Verification items for the finished model (mm, model axes). A direction names the side the tool comes from. Give positions to 0.01 mm unless a question says otherwise; leave off trailing zeros. Order: outer loops, then holes, each group sorted by start corner. A loop starts at its lowest first (then second) coordinate and runs counter-clockwise, first axis right, second up.
from build123d import *

# Parameters (mm, degrees)
F0_W      = 12.7
F0_H      = 6.35
F1_DEPTH  = 12.7
F2_R      = 5.08
F3_W      = 6.35
F3_H      = 8.89
F4_DEPTH  = 12.7
F6_DEPTH  = 5.715
F7_W      = 3.81
F7_H      = 12.7
F8_DEPTH  = 12.7
F10_DEPTH = 25.4


with BuildPart() as f1:
    # F0 (on Front) → F1 (new body)
    with BuildSketch(Plane.XZ):
        Polygon((-6.35, -3.175), (-6.35, 3.175), (-12.0512209833, 3.175), (-12.0512209833, -15.875), (-6.35, -15.875), align=None)
        Rectangle(F0_W, F0_H)
        Polygon((12.4626047909, 3.175), (6.35, 3.175), (6.35, -3.175), (6.35, -15.875), (12.4626047909, -15.875), align=None)
    extrude(amount=F1_DEPTH)

    # F2
    f2_edges = [f1.edges().sort_by_distance(p)[0] for p in [
        (-12.051221, -6.35, 3.175),
        (12.462605, -6.35, 3.175),
        (-12.051221, -6.35, -15.875),
        (12.462605, -6.35, -15.875),
    ]]
    fillet(f2_edges, radius=F2_R)

    # F3 (on face) → F4 (cut)
    with BuildSketch(Plane.YZ.offset(12.4626047909)):
        with Locations((-6.35, -6.35)):
            Rectangle(F3_W, F3_H)
        with Locations((-6.35, -15.24)):
            Rectangle(F3_W, F3_H)
    extrude(amount=-F4_DEPTH, mode=Mode.SUBTRACT)

    # F5 (on face) → F6 (join)
    with BuildSketch(Plane.YZ.offset(12.4626047909)):
        with BuildLine():
            Line((-6.35, -4.445), (-6.35, -1.905))
            Line((-6.35, -1.905), (-9.525, -1.905))
            add(Edge.make_bspline(
                [(-9.525, -1.905), (-6.35, -1.905), (-7.4083333333, -3.5983333333), (-6.35, -4.445)],
                knots=[0, 0, 0, 0, 4.0659838908, 4.0659838908, 4.0659838908, 4.0659838908], degree=3))
        make_face()
        with BuildLine():
            add(Edge.make_bspline(
                [(-3.175, -1.905), (-6.35, -1.905), (-5.2916666667, -3.5983333333), (-6.35, -4.445)],
                knots=[0, 0, 0, 0, 4.0659838908, 4.0659838908, 4.0659838908, 4.0659838908], degree=3))
            Line((-3.175, -1.905), (-6.35, -1.905))
            Line((-6.35, -1.905), (-6.35, -4.445))
        make_face()
    extrude(amount=-F6_DEPTH)

    # F7 (on face) → F8 (join)
    with BuildSketch(Plane.XY.offset(3.175)):
        with Locations((0, -6.35)):
            Rectangle(F7_W, F7_H)
    extrude(amount=F8_DEPTH)

    # F9 (on face) → F10 (cut)
    with BuildSketch(Plane.YZ.offset(1.905)):
        with BuildLine():
            Line((-12.7, 15.875), (-12.7, 3.175))
            add(Edge.make_bspline(
                [(-12.7, 3.175), (-6.35, 3.175), (-12.7, 3.175), (-6.35, 15.875)],
                knots=[0, 0, 0, 0, 14.1990316571, 14.1990316571, 14.1990316571, 14.1990316571], degree=3))
            Line((-6.35, 15.875), (-12.7, 15.875))
        make_face()
        with BuildLine():
            Line((0, 15.875), (-6.35, 15.875))
            add(Edge.make_bspline(
                [(-6.35, 15.875), (0, 3.175), (-6.35, 3.175), (0, 3.175)],
                knots=[0, 0, 0, 0, 14.1990316571, 14.1990316571, 14.1990316571, 14.1990316571], degree=3))
            Line((0, 3.175), (0, 15.875))
        make_face()
    extrude(amount=-F10_DEPTH, mode=Mode.SUBTRACT)


solid = f1.part
(1) Section check C-C, the plane z = -13. Enter the section's corners in (x, y) (3 decimals), then the cut area to 3 significant figures.
Solved:
outline: (-11.548, -12.7) - (-6.35, -12.7) - (-6.35, 0) - (-11.548, 0) - close; (6.35, -12.7) - (11.959, -12.7) - (11.959, -9.525) - (6.35, -9.525) - close; (6.35, -3.175) - (11.959, -3.175) - (11.959, 0) - (6.35, 0) - close
area: 102 mm2
(2) Section check D-D, the plane x = -5.75. Enter the section's corners in (y, z) (3 decimals), then the cut area to 3 significant figures.
Solved:
outline: (-12.7, -3.175) - (0, -3.175) - (0, 3.175) - (-12.7, 3.175) - close
area: 80.6 mm2
(3) Go/stop test with flat-tipped pins: pin 1 (2.5 mm diameter, centred on x = -5, y = -4.5, fed in from +Z) (3 decimals); pin 2 (3 mm diameter, centred on x = 3, y = -5, fed in from -Z) (3 decimals); pin 3 (4 mm diameter, centred on y = -3.5, z = -7, fed in from +X); pin 4 (2 mm diameter, centred on y = -7.5, z = 6, fed in from -X) (3 decimals). Record where each tip stops, or that it passes through.
Solved:
pin 1: stops at z = 3.175
pin 2: stops at z = -1.905
pin 3: stops at x = 12.46
pin 4: stops at x = -1.905
(4) Section check A-A, the plane z = -7.5. Enter the section's corners in (x, y) (3 decimals).
Solved:
outline: (-12.051, -12.7) - (-6.35, -12.7) - (-6.35, 0) - (-12.051, 0) - close; (6.35, -12.7) - (12.463, -12.7) - (12.463, -9.525) - (6.35, -9.525) - close; (6.35, -3.175) - (12.463, -3.175) - (12.463, 0) - (6.35, 0) - close
(5) Section check B-B, the plane x = 4.5. Enter the section's corners in (y, z) (3 decimals), then the cut area to 3 significant figures.
Solved:
outline: (-12.7, -3.175) - (-9.525, -3.175) - (-9.525, -1.905) - (-3.175, -1.905) - (-3.175, -3.175) - (0, -3.175) - (0, 3.175) - (-12.7, 3.175) - close
area: 72.6 mm2
(6) Set-up check for faces 5 (the flat face through (6.748, -6, -3)), 6 (the flat face through (9, -3.175, -7)), 7 (the flat face through (-6.35, -6, -10)), 8 (the flat face through (5, -6, 3.175)): record each of +Z, -Z, +X, -X, +Y, -Y from which the full face is reachable in a straight line by a thin tool's end or side.
Solved:
face 5: -Z
face 6: -Z, +X
face 7: -Z, +Y, -Y
face 8: +Z, +X, +Y, -Y
(7) Release check for a two-part mould opening along X. For faces 1 (the flat face through (6.35, -2, -9)), 2 (the flat face through (9, -9.525, -7)), 3 (the flat face through (3, -6, -1.905)), 4 (the flat face through (-12.051, -6, -6)) record: pulls with the +X half, pulls with the -X half, needs draft (parallel to the pull), parting line crosses it, or undercut.
Solved:
face 1: undercut
face 2: needs draft
face 3: undercut
face 4: pulls with the -X half
(8) Scan lines: line 1 (Y direction, x = 9.75, z = -5) (3 decimals); line 2 (X direction, y = -4, z = -10.5); line 3 (Z direction, x = 4.75, y = -2.75) (3 decimals). Record each from-to range of solid material in increasing order.
Solved:
line 1: y = -12.7 to -9.525, -3.175 to 0
line 2: x = -12.05 to -6.35
line 3: z = -3.175 to 3.175
